from build123d import *

# Parameters (mm, degrees)
F1_DEPTH  = 38.1
F2_R      = 9.525
F3_DEPTH  = 50.8
F5_R      = 9.525
F6_DEPTH  = 44.45
F8_DEPTH  = 46.482
F10_DEPTH = 38.1
F11_R     = 1.5875
F12_DEPTH = 57.15


with BuildPart() as f1:
    # F0 (on Front) → F1 (new body)
    with BuildSketch(Plane.XZ):
        Polygon((0, 63.5), (0, 0), (304.8, 0), (304.8, 19.05), align=None)
    extrude(amount=F1_DEPTH)

    # F2 (on face) → F3 (join)
    with BuildSketch(Plane(origin=(0, 0, 0), x_dir=(0, -1, 0), z_dir=(-1, 0, 0))):
        with Locations((19.05, 31.75)):
            Circle(F2_R)
    extrude(amount=-F3_DEPTH)

    # F5 (on face) → F6 (cut)
    with BuildSketch(Plane(origin=(0, 0, 0), x_dir=(0, -1, 0), z_dir=(-1, 0, 0))):
        with Locations((19.05, 31.75)):
            Circle(F5_R)
    extrude(amount=-F6_DEPTH, mode=Mode.SUBTRACT)

    # F7 (on face) → F8 (cut)
    with BuildSketch(Plane.XZ.offset(38.1)):
        with BuildLine():
            Line((0, 63.5), (0, 44.45))
            Line((0, 44.45), (64.008, 44.45))
            ThreePointArc((64.008, 44.45), (71.925847, 40.815134), (74.330844, 32.441333))
            Line((74.330844, 32.441333), (304.799885, 17.554725))
            Line((304.799885, 17.554725), (304.799885, 0))
            Line((304.799885, 0), (304.8, 0))
            Line((304.8, 0), (304.8, 19.05))
            Line((304.8, 19.05), (0, 63.5))
        make_face()
    extrude(amount=-F8_DEPTH, mode=Mode.SUBTRACT)

    # F9 (on face) → F10 (cut)
    with BuildSketch(Plane(origin=(2.395601, 0, 37.087822), x_dir=(0.99792, 0, -0.064458), z_dir=(0.064458, 0, 0.99792))):
        Polygon((303.034474, -19.05), (290.334474, -6.35), (74.434474, -6.35), (74.434474, -31.75), (290.334474, -31.75), align=None)
    extrude(amount=-F10_DEPTH, mode=Mode.SUBTRACT)

    # F11 (on face) → F12 (cut)
    with BuildSketch(Plane.XZ.offset(38.1)):
        with Locations((34.718972, 10.036203)):
            Circle(F11_R)
        with Locations((299.694479, 8.33375)):
            Circle(F11_R)
    extrude(amount=-F12_DEPTH, mode=Mode.SUBTRACT)


solid = f1.part
Read the model definition and answer for the solid it produces. Units are mm, in the model's axes. A direction names the side the tool comes from. Round coordinates to 2 decimals unless told otherwise and drop trailing zeros. Loops run counter-clockwise (first coordinate to the right, second up) from the corner with the lowest first, then second, coordinate; pieces in that order, holes last. Notation, with made-up numbers: (58, 81) - (63, 81) arc R31 cw to (63, 106) - close; hole circle Ø8 at (-27, 57.25). An arc over 180 degrees is marked (long way). One line per question, with ' | ' between items. Start each with the question number.
Q1. Find the intervals of material crossed by L1, parallel to Z at x = 36, y = -12; L2, parallel to Y at x = 27, z = 32; L3, parallel to Y at x = 168.5, z = 5, in increasing order.
Q2. Section C-C on x = 85 is taken. Give the vertices of the cut face in (y, z).
Q3. For faces 4 (the flat face through (297.79, -25.49, 8.91)), 5 (the flat face through (116, 0, 18)), 6 (the flat face through (32, -19, 44.45)), 7 (the cylindrical face through (21.91, -16.99, 22.45)), 8 (the flat face through (182, -31.75, 13)), determine the directions among +Z, -Z, +X, -X, +Y, -Y from which every point of the face is accessible in a straight line to the end or side of a thin tool.
Q4. For a pull along X with two mould halves and no side action, classify faces 1 (the flat face through (75.647, -18.872, 16.371)), 2 (the flat face through (116, -6, 0)), 3 (the flat face through (0, -19, 18)) as +X half, -X half, draft (parallel to the pull), parting line (faces both ways), or undercut.
Q5. Flat-ended cylindrical pins translate along their axes: pin 1 (12 mm diameter, centred on y = -13, z = 36, fed in from +X); pin 2 (4 mm diameter, centred on x = 299.69, z = 8.33, fed in from -Y); pin 3 (5 mm diameter, centred on x = 96.5, y = -28.5, fed in from -Z); pin 4 (1 mm diameter, centred on x = 211, y = -34, fed in from +Z). Find the tip coordinate at first contact, or state that the pin passes through.
Q6. Section A-A on x = 146.5 is taken. Give the vertices of the cut face in (y, z), plus the area to 3 significant figures.
Q7. Section B-B on z = 28.5 is taken. Give the vertices of the cut face in (x, y), plus the area to 3 significant figures.
Established:
1) L1: 0 to 9.1, 10.97 to 25.35, 38.15 to 44.45 | L2: -38.1 to -28.57, -9.53 to 0 | L3: -38.1 to -31.75, -6.35 to 0
2) outline: (-38.1, 0) - (-31.75, 0) - (-31.75, 31.75) - (-38.1, 31.75) - close; (-6.35, 0) - (0, 0) - (0, 31.75) - (-6.35, 31.75) - close
3) face 4: +Z | face 5: +Z, -Z, +X, -X, +Y | face 6: +Z, +X, -X, +Y, -Y | face 7: -X | face 8: +Z, -Z
4) face 1: undercut | face 2: draft | face 3: -X half
5) pin 1: x = 76.68 | pin 2: y = -38.1 | pin 3: through | pin 4: z = 23.65
6) outline: (-38.1, 0) - (-31.75, 0) - (-31.75, 27.78) - (-38.1, 27.78) - close; (-6.35, 0) - (0, 0) - (0, 27.78) - (-6.35, 27.78) - close | area: 353 mm²
7) outline: (0, -38.1) - (135.35, -38.1) - (135.35, -31.75) - (76.43, -31.75) - (76.43, -6.35) - (135.35, -6.35) - (135.35, 0) - (0, 0) - (0, -10.1) - (44.45, -10.1) - (44.45, -28) - (0, -28) - close | area: 2,860 mm²
